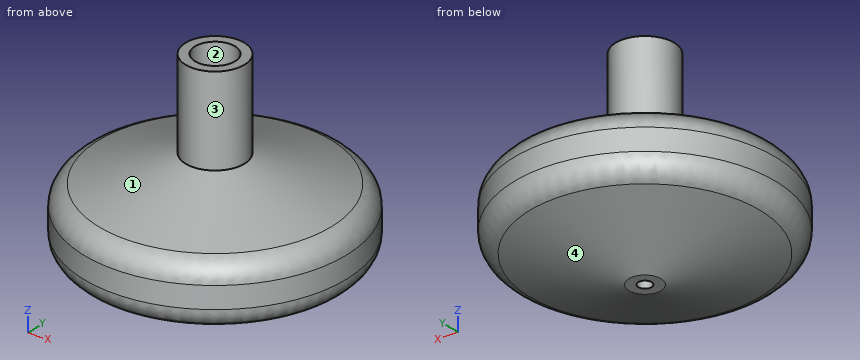
```python
from build123d import *

# Parameters (mm, degrees)
F2_R     = 4.7625
F3_DEPTH = 9.525
F4_R     = 1.5875
F5_DEPTH = 22.225
F6_R     = 5.08


with BuildPart() as f1:
    # F0 (on Front) → F1 (revolve)
    with BuildSketch(Plane.XZ):
        Polygon((3.81, 1.888357), (31.115, 9.508357), (31.115, 22.208357), (6.985, 29.828357), (6.985, 50.8), (0, 50.8), (0, 1.888357), align=None)
    revolve(axis=Axis((0, 0, 26.344178), (0, 0, -1)))

    # F2 (on face) → F3 (cut)
    with BuildSketch(Plane.XY.offset(50.8)):
        Circle(F2_R)
    extrude(amount=-F3_DEPTH, mode=Mode.SUBTRACT)

    # F4 (on face) → F5 (cut)
    with BuildSketch(Plane(origin=(0, 0, 1.888357), x_dir=(1, 0, 0), z_dir=(0, 0, -1))):
        Circle(F4_R)
    extrude(amount=-F5_DEPTH, mode=Mode.SUBTRACT)

    # F6
    f6_edges = [f1.edges().sort_by_distance(p)[0] for p in [
        (-31.115, 0, 9.508357),
        (-31.115, 0, 22.208357),
        (31.115, 0, 15.858357),
    ]]
    fillet(f6_edges, radius=F6_R)


solid = f1.part
```
The listing builds one solid part. Answer for the finished solid, in the listing's coordinates (mm). Face numbers are marked on the shaded views. A direction names the side the tool comes from. Coordinates: 2 decimals unless noted, no trailing zeros. Loops run counter-clockwise (first coordinate to the right, second up) from the corner with the lowest first, then second, coordinate; pieces in that order, holes last. Notation, with made-up numbers: (39.25, -18) -> (48.25, -18) arc R32 ccw to (48.25, 10) -> close; hole circle Ø1 at (-17, 65.5). An arc over 180 degrees is marked (long way). Use one line per item in the form item = value. Start each with the question number.
Item 1: Consider L1, parallel to Y at x = 0, z = 48 (1 decimal); L2, parallel to X at y = 0, z = 15.25 (1 decimal); L3, parallel to X at y = -2.5, z = 44. Determine where each line is inside the solid, lowest interval first. Write a range as [from, to].
Item 2: The part is cut by section C-C on z = 26.5. Determine the outline of the cut face in (x, y), then the cut area to 3 significant figures.
Item 3: The part is cut by section B-B on z = 38. Determine the outline of the cut face in (x, y) (3 decimals).
Item 4: The mould has two halves that part along Y. Classify the marked faces 1 and 2: released by +Y, released by -Y, zero draft, split by the parting line, or undercut.
Item 5: The part is cut by section A-A on z = 48. Determine the outline of the cut face in (x, y) (1 decimal).
Item 6: A tool of negligible diameter and unlimited length cuts with its end or side. For the marked faces 3 and 4, from which of +Z, -Z, +X, -X, +Y, -Y can it reach the whole face along a straight path? Write none if from no direction.
Item 7: Flat-ended cylindrical pins translate along their axes: pin 1 Ø1 at (x, z) = (-16.5, 23) entering from +Y; pin 2 Ø10 at (x, y) = (15, -14.5) entering from -Z; pin 3 Ø3 at (x, y) = (1.5, -1.5) entering from +Z (3 decimals). Find the tip coordinate at first contact, or state that the pin passes through.
Answer key:
q1.L1 = [-7, -4.8], [4.8, 7]
q1.L2 = [-31.1, -1.6], [1.6, 31.1]
q1.L3 = [-6.52, -4.05], [4.05, 6.52]
q2.outline = circle Ø35.05 at (0, 0)
q2.area = 965 mm2
q3.outline = circle Ø13.97 at (0, 0)
q4.face_1 = split by the parting line
q4.face_2 = undercut
q5.outline = circle Ø14 at (0, 0); hole circle Ø9.5 at (0, 0)
q6.face_3 = +Z
q6.face_4 = -Z
q7.pin_1 = 24.1
q7.pin_2 = 5.25
q7.pin_3 = 41.275
